Could you check a few things on this model? Use its own coordinates, in mm. Face numbers are marked on the shaded views. A direction names the side the tool comes from. Give positions to 0.01 mm unless a question says otherwise; leave off trailing zeros. Write each loop counter-clockwise with the first axis right and the second up, starting at its lowest first coordinate (ties: lowest second). Pieces come first, ordered by that corner, then holes. Notation, with made-up numbers: M 26.5,39.5 L 32.5,39.5 A20 ccw 32.5,57.5 Z; hole C 12,-36.5 d9. An arc over 180 degrees is marked long. Answer as CSV lines item,"result". Start each with the question number.
Autodesk Inventor part; units mm, degrees
ref_plane "YZ Plane" through (0, 0, 0) normal (1, 0, 0) x (0, 1, 0)
ref_plane "XZ Plane" through (0, 0, 0) normal (0, 1, 0) x (-1, 0, 0)
ref_plane "XY Plane" through (0, 0, 0) normal (0, 0, 1) x (1, 0, 0)
sketch "スケッチ1" plane through (0, 0, 0) normal (1, 0, 0) x (0, 1, 0)
  circle A0 centre (0, 0) radius 7.5
  dimension "d0" = 15
extrude "押し出し1" add sketch "スケッチ1" along normal blind 4
sketch "スケッチ2" plane through (0, 0, 0) normal (0, 1, 0) x (-1, 0, 0)
  circle A0 centre (8.5, 0) radius 2
  circle A1 centre (8.5, 0) radius 3
  line L0 (8.5, -3) -> (0, -3)
  line L1 (0, 7.5) -> (0, -7.5)
  line L2 (8.5, 3) -> (0, 3)
  point P0 (0, 0)
  dimension "d3" = 4
  dimension "d4" = 6
  dimension "d5" = 8.5
extrude "押し出し2" add sketch "スケッチ2" along normal mid plane 4
sketch "スケッチ3" plane through (4, 0, 0) normal (1, 0, 0) x (0, 0, -1)
  circle A0 centre (0, 0) radius 2
  dimension "d8" = 4
extrude "押し出し3" add sketch "スケッチ3" along normal blind 10
properties part number "pink-suspension-top" material "ABS プラスチック"
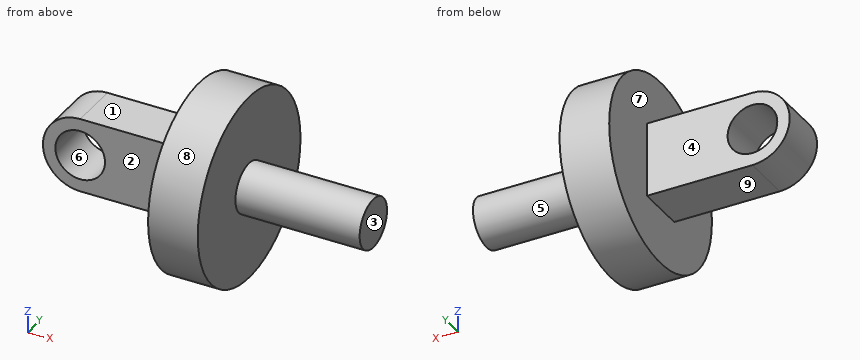
1. Please list where these lines run through material, in increasing order: line 1 (X direction, y = -4.25, z = -6); line 2 (Y direction, x = -7, z = 2.75); line 3 (Y direction, x = 1.25, z = 3).
2. Imagine slicing it at A-A, the plane y = 0. Please give me the cut outline in (x, z), plus the area to 3 significant figures.
3. Will these pins go through, and if not, where does the flat tip stop? P1, Ø3, axis at x = -7.5, z = -1.5, coming from the +Y side; P2, Ø2, axis at x = -6, z = 0, coming from the -Y side; P3, Ø1, axis at x = 8, z = 2, coming from the +Y side.
4. Imagine slicing it at D-D, the plane z = -5.75. Please give me the cut outline in (x, y).
5. Imagine slicing it at B-B, the plane z = 0. Please give me the cut outline in (x, y), plus the area to 3 significant figures.
6. Imagine slicing it at C-C, the plane x = 5.75. Please give me the cut outline in (y, z), plus the area to 3 significant figures.
7. Thinking about a two-plate mould opening in Z: for the marked faces 6, 7, 8 and 9, which applies, pulls with the +Z half, pulls with the -Z half, needs draft (parallel to the pull), parting line crosses it, or undercut?
8. On a 3-axis mill with a long thin cutter (end or side, diameter ignored), from which of +Z, -Z, +X, -X, +Y, -Y can I reach the whole of each face in a straight line? I mean the marked faces 1, 2, 3, 4 and 5. Say none if no direction works.
Solutions:
1,line 1,"0 to 4"
1,line 2,"-2 to 2"
1,line 3,"-6.87 to 6.87"
2,outline,"M -8.5,-3 L 0,-3 L 0,-7.5 L 4,-7.5 L 4,-2 L 14,-2 L 14,2 L 4,2 L 4,7.5 L 0,7.5 L 0,3 L -8.5,3 A3 ccw Z; hole C -8.5,0 d4"
2,area,"153 mm²"
3,P1,"y = 2"
3,P2,"y = -2"
3,P3,"y = 1.32"
4,outline,"M 0,-4.82 L 4,-4.82 L 4,4.82 L 0,4.82 Z"
5,outline,"M -11.5,-2 L -10.5,-2 L -10.5,2 L -11.5,2 Z; M -6.5,-2 L 0,-2 L 0,-7.5 L 4,-7.5 L 4,-2 L 14,-2 L 14,2 L 4,2 L 4,7.5 L 0,7.5 L 0,2 L -6.5,2 Z"
5,area,"130 mm²"
6,outline,"C 0,0 d4"
6,area,"12.6 mm²"
7,face 6,"undercut"
7,face 7,"needs draft"
7,face 8,"parting line crosses it"
7,face 9,"pulls with the -Z half"
8,face 1,"+Z, -X, +Y, -Y"
8,face 2,"+Z, -Z, -X, -Y"
8,face 3,"+Z, -Z, +X, +Y, -Y"
8,face 4,"+Z, -Z, -X, +Y"
8,face 5,"+X"
